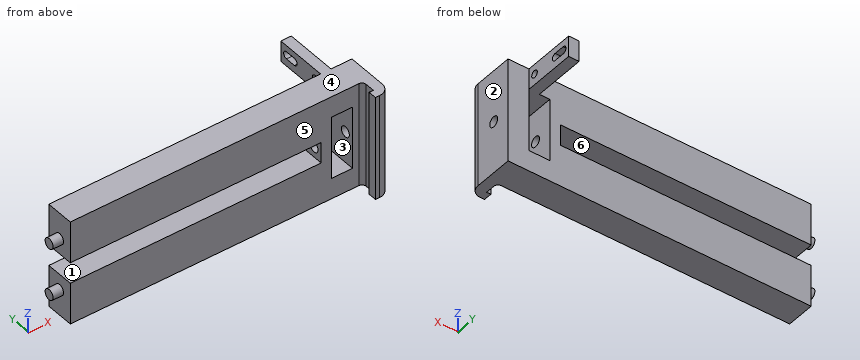
from build123d import *

# Parameters (mm, degrees)
SKETCH1_W               = 140
SKETCH1_H               = 13.5
BOSS_EXTRUDE1_DEPTH     = 50
SKETCH2_R               = 2.5
BOSS_EXTRUDE2_DEPTH     = 5
SKETCH6_W               = 50
SKETCH6_H               = 24
BOSS_EXTRUDE4_DEPTH     = 5
CUT_EXTRUDE1_DEPTH      = 156.244967712
CUT_EXTRUDE1_DEPTH_BACK = 156.244967712
SKETCH4_W               = 10
SKETCH4_H               = 30
SKETCH7_R               = 2.5
CUT_EXTRUDE3_DEPTH      = 35
SKETCH8_W               = 50
SKETCH8_H               = 4
BOSS_EXTRUDE5_DEPTH     = 2
SKETCH9_W               = 120
SKETCH9_H               = 10
CUT_EXTRUDE4_DEPTH      = 15
SKETCH10_W              = 5
SKETCH10_H              = 10
BOSS_EXTRUDE6_DEPTH     = 25
CUT_EXTRUDE5_DEPTH      = 150.020971678
CUT_EXTRUDE5_DEPTH_BACK = 150.020971678
SKETCH13_R              = 1.75
FILLET1_R               = 2
FILLET2_R               = 5


with BuildPart() as part:
    # Sketch1 → Boss-Extrude1 (new body)
    with BuildSketch(Plane.XY):
        with Locations((-70, 6.75)):
            Rectangle(SKETCH1_W, SKETCH1_H)
    extrude(amount=BOSS_EXTRUDE1_DEPTH)

    # Sketch2 → Boss-Extrude2 (add)
    with BuildSketch(Plane.ZY.offset(140)):
        with Locations(Location((12.5, 6.75, 0), (0, 0, 180))):
            Circle(SKETCH2_R)
        with Locations(Location((37.5, 6.75, 0), (0, 0, 180))):
            Circle(SKETCH2_R)
    extrude(amount=BOSS_EXTRUDE2_DEPTH)

    # Sketch6 → Boss-Extrude4 (add)
    with BuildSketch(Plane(origin=(0, 0, 0), x_dir=(0, 0, -1), z_dir=(1, 0, 0))):
        with Locations((-25, 1.5)):
            Rectangle(SKETCH6_W, SKETCH6_H)
    extrude(amount=BOSS_EXTRUDE4_DEPTH)

    # Sketch4 → Cut-Extrude1 (cut, two sides: drawn at the far end of the back side and taken through both)
    with BuildSketch(Plane(origin=(0, 13.5, 0), x_dir=(1, 0, 0), z_dir=(0, 1, 0)).offset(-CUT_EXTRUDE1_DEPTH_BACK)):
        with Locations((-10, -25)):
            Rectangle(SKETCH4_W, SKETCH4_H)
    extrude(amount=CUT_EXTRUDE1_DEPTH + CUT_EXTRUDE1_DEPTH_BACK, mode=Mode.SUBTRACT)

    # Sketch7 → Cut-Extrude3 (cut)
    with BuildSketch(Plane(origin=(5, 0, 0), x_dir=(0, 0, -1), z_dir=(1, 0, 0))):
        with Locations(Location((-25, 4.5, 0), (0, 0, 90))):
            Circle(SKETCH7_R)
    extrude(amount=-CUT_EXTRUDE3_DEPTH, mode=Mode.SUBTRACT)

    # Sketch8 → Boss-Extrude5 (add)
    with BuildSketch(Plane.ZY):
        with Locations((25, -8.5)):
            Rectangle(SKETCH8_W, SKETCH8_H)
    extrude(amount=BOSS_EXTRUDE5_DEPTH)

    # Sketch9 → Cut-Extrude4 (cut)
    with BuildSketch(Plane(origin=(0, 13.5, 0), x_dir=(1, 0, 0), z_dir=(0, 1, 0))):
        with Locations((-80, -25)):
            Rectangle(SKETCH9_W, SKETCH9_H)
    extrude(amount=-CUT_EXTRUDE4_DEPTH, mode=Mode.SUBTRACT)

    # Sketch10 → Boss-Extrude6 (add)
    with BuildSketch(Plane(origin=(0, 13.5, 0), x_dir=(1, 0, 0), z_dir=(0, 1, 0))):
        with Locations((-7.5, -45)):
            Rectangle(SKETCH10_W, SKETCH10_H)
    extrude(amount=BOSS_EXTRUDE6_DEPTH)

    # Sketch13 → Cut-Extrude5 (cut, two sides: drawn at the far end of the back side and taken through both)
    with BuildSketch(Plane.ZY.offset(10).offset(-CUT_EXTRUDE5_DEPTH_BACK)):
        with Locations((45.25, 17)):
            Circle(SKETCH13_R)
        with BuildLine():
            Line((43.5, 30), (43.5, 35))
            ThreePointArc((43.5, 35), (45.25, 36.75), (47, 35))
            Line((47, 35), (47, 30))
            ThreePointArc((47, 30), (45.25, 28.25), (43.5, 30))
        make_face()
    extrude(amount=CUT_EXTRUDE5_DEPTH + CUT_EXTRUDE5_DEPTH_BACK, mode=Mode.SUBTRACT)

    # Fillet1
    fillet1_edges = [part.edges().sort_by_distance(p)[0] for p in [
        (0, 0, 25),
    ]]
    fillet(fillet1_edges, radius=FILLET1_R)

    # Fillet2
    fillet2_edges = [part.edges().sort_by_distance(p)[0] for p in [
        (5, -10.5, 25),
    ]]
    fillet(fillet2_edges, radius=FILLET2_R)


solid = part.part
Geometry: final body of the model. Coordinates: model frame, mm. Face numbers are marked on the shaded views. A direction names the side the tool comes from. Give positions to 0.01 mm unless a question says otherwise; leave off trailing zeros. Write each loop counter-clockwise with the first axis right and the second up, starting at its lowest first coordinate (ties: lowest second). Pieces come first, ordered by that corner, then holes. Notation, with made-up numbers: (-38.5, -17) -> (14.5, -17) arc R21 ccw to (14.5, 22) -> close; hole circle Ø10 at (30, 7). An arc over 180 degrees is marked (long way). Answer in a Markdown table with one row per item.
(1) Section query B-B on x = -45. Return loops of the section in (y, z), then the cut area to 3 significant figures.
Answers below:
| item | result |
|---|---|
| outline | (0, 0) -> (13.5, 0) -> (13.5, 20) -> (0, 20) -> close; (0, 30) -> (13.5, 30) -> (13.5, 50) -> (0, 50) -> close |
| area | 540 mm^2 |
(2) Section query D-D on z = 37.5. Return loops of the section in (x, y), then the cut area to 3 significant figures.
Answers below:
| item | result |
|---|---|
| outline | (-145, 4.25) -> (-140, 4.25) -> (-140, 0) -> (-15, 0) -> (-15, 13.5) -> (-140, 13.5) -> (-140, 9.25) -> (-145, 9.25) -> close; (-5, 0) -> (-2, 0) arc R2 cw to (0, -2) -> (0, -6.5) -> (-2, -6.5) -> (-2, -10.5) -> (0, -10.5) arc R5 ccw to (5, -5.5) -> (5, 13.5) -> (-5, 13.5) -> close |
| area | 1,900 mm^2 |
(3) Ray query, line 1 along Y through (x, z) = (-8.4, 45.25); line 2 along X through (y, z) = (11, 29); line 3 along X through (y, z) = (1, 38). Return the intervals inside material, ascending. Write a range as [from, to].
Answers below:
| item | result |
|---|---|
| line 1 | [0, 15.25], [18.75, 28.25], [36.75, 38.5] |
| line 2 | [-20, -15], [-5, 5] |
| line 3 | [-140, -15], [-5, 5] |
(4) Section query A-A on z = 45.25. Return loops of the section in (x, y), then the cut area to 3 significant figures.
Answers below:
| item | result |
|---|---|
| outline | (-140, 0) -> (-2, 0) arc R2 cw to (0, -2) -> (0, -6.5) -> (-2, -6.5) -> (-2, -10.5) -> (0, -10.5) arc R5 ccw to (5, -5.5) -> (5, 13.5) -> (-5, 13.5) -> (-5, 15.25) -> (-10, 15.25) -> (-10, 13.5) -> (-140, 13.5) -> close; (-10, 18.75) -> (-5, 18.75) -> (-5, 28.25) -> (-10, 28.25) -> close; (-10, 36.75) -> (-5, 36.75) -> (-5, 38.5) -> (-10, 38.5) -> close |
| area | 2,080 mm^2 |
(5) Set-up query: the marked faces 1, 2 and 3. Return all of +Z, -Z, +X, -X, +Y, -Y with unobstructed straight access to the full face (end or side cutting, diameter ignored); none if empty.
Answers below:
| item | result |
|---|---|
| face 1 | -X, +Y, -Y |
| face 2 | +Z, -Z, +X, +Y, -Y |
| face 3 | +Y, -Y |
(6) Section query C-C on y = 12. Return loops of the section in (x, z).
Answers below:
| item | result |
|---|---|
| outline | (-140, 0) -> (5, 0) -> (5, 50) -> (-140, 50) -> (-140, 30) -> (-20, 30) -> (-20, 20) -> (-140, 20) -> close; hole (-15, 10) -> (-5, 10) -> (-5, 40) -> (-15, 40) -> close |
(7) Pin query (flat end, axial travel): pin 1 (1.3 mm diameter, centred on y = -5, z = 28.5, fed in from -X); pin 2 (3 mm diameter, centred on y = 21.5, z = 46, fed in from -X); pin 3 (10 mm diameter, centred on x = -96.5, z = 7.5, fed in from -Y). Return the tip coordinate at first contact, or that it passes through.
Answers below:
| item | result |
|---|---|
| pin 1 | x = 0 |
| pin 2 | x = -10 |
| pin 3 | y = 0 |
(8) Draft query along Z for the marked faces 4, 5 and 6. Return one class per face: +Z half, -Z half, draft (parallel to the pull), parting line (faces both ways), or undercut.
Answers below:
| item | result |
|---|---|
| face 4 | +Z half |
| face 5 | draft |
| face 6 | undercut |
